The model under review builds one solid part; all positions refer to its coordinate system, in mm. A direction names the side the tool comes from. Round coordinates to 2 decimals unless told otherwise and drop trailing zeros. Order: outer loops, then holes, each group sorted by start corner. A loop starts at its lowest first (then second) coordinate and runs counter-clockwise, first axis right, second up. Notation, with made-up numbers: M 76.25,82 L 115.25,82 A22 ccw 115.25,109 Z; hole C 51.25,68.25 d9. An arc over 180 degrees is marked long. Answer as CSV lines item,"result". Start each with the question number.
from build123d import *

# Parameters (mm, degrees)
SKETCH_1_W          = 140
SKETCH_1_H          = 75
EXTRUDE_1_DEPTH     = 3
SKETCH_2_R          = 1.55
CUT_EXTRUDE_1_DEPTH = 3
SKETCH_3_W          = 5
SKETCH_3_H          = 55
EXTRUDE_2_DEPTH     = 15
SKETCH_5_R          = 1.55
CUT_EXTRUDE_2_DEPTH = 15
SKETCH_6_R          = 1.55
CUT_EXTRUDE_3_DEPTH = 15
FILLET_1_R          = 2
FILLET_2_R          = 1


with BuildPart() as part:
    # 草图1 → 凸台-拉伸1 (new body)
    with BuildSketch(Plane(origin=(0, 0, 0), x_dir=(1, 0, 0), z_dir=(0, 1, 0))):
        Rectangle(SKETCH_1_W, SKETCH_1_H)
    extrude(amount=EXTRUDE_1_DEPTH)

    # 草图2 → 切除-拉伸1 (cut)
    with BuildSketch(Plane.XZ):
        with Locations(Location((-49, 0, 0), (0, 0, 270))):
            Circle(SKETCH_2_R)
        with Locations(Location((-49, -30, 0), (0, 0, 270))):
            Circle(SKETCH_2_R)
        with Locations(Location((-49, 30, 0), (0, 0, 270))):
            Circle(SKETCH_2_R)
        with Locations(Location((49, 30, 0), (0, 0, 270))):
            Circle(SKETCH_2_R)
        with Locations(Location((49, 0, 0), (0, 0, 270))):
            Circle(SKETCH_2_R)
        with Locations(Location((49, -30, 0), (0, 0, 270))):
            Circle(SKETCH_2_R)
    extrude(amount=-CUT_EXTRUDE_1_DEPTH, mode=Mode.SUBTRACT)

    # 草图3 → 凸台-拉伸2 (add)
    with BuildSketch(Plane.XZ):
        with Locations((-59.5, 0)):
            Rectangle(SKETCH_3_W, SKETCH_3_H)
        with Locations((59.5, 0)):
            Rectangle(SKETCH_3_W, SKETCH_3_H)
    extrude(amount=EXTRUDE_2_DEPTH)

    # 草图5 → 切除-拉伸2 (cut)
    with BuildSketch(Plane.XZ):
        with Locations(Location((-66, 20, 0), (0, 0, 270))):
            Circle(SKETCH_5_R)
        with Locations(Location((-66, 10, 0), (0, 0, 270))):
            Circle(SKETCH_5_R)
        with Locations(Location((-66, 0, 0), (0, 0, 270))):
            Circle(SKETCH_5_R)
        with Locations(Location((-66, -10, 0), (0, 0, 270))):
            Circle(SKETCH_5_R)
        with Locations(Location((-66, -20, 0), (0, 0, 270))):
            Circle(SKETCH_5_R)
        with Locations(Location((66, -20, 0), (0, 0, 270))):
            Circle(SKETCH_5_R)
        with Locations(Location((66, -10, 0), (0, 0, 270))):
            Circle(SKETCH_5_R)
        with Locations(Location((66, 0, 0), (0, 0, 270))):
            Circle(SKETCH_5_R)
        with Locations(Location((66, 10, 0), (0, 0, 270))):
            Circle(SKETCH_5_R)
        with Locations(Location((66, 20, 0), (0, 0, 270))):
            Circle(SKETCH_5_R)
    extrude(amount=-CUT_EXTRUDE_2_DEPTH, mode=Mode.SUBTRACT)

    # 草图6 → 切除-拉伸3 (cut)
    with BuildSketch(Plane.ZY.offset(62)):
        with Locations((-20.625, -12.5)):
            Circle(SKETCH_6_R)
        with Locations((-13.766824394, -12.463345811)):
            Circle(SKETCH_6_R)
        with Locations((-6.911518496, -12.401024848)):
            Circle(SKETCH_6_R)
        with Locations((6.736772336, -12.494506292)):
            Circle(SKETCH_6_R)
        with Locations((13.810201603, -12.556827255)):
            Circle(SKETCH_6_R)
        with Locations((20.572026056, -12.587987736)):
            Circle(SKETCH_6_R)
    cut_extrude_3 = extrude(amount=-CUT_EXTRUDE_3_DEPTH, mode=Mode.SUBTRACT)

    # 镜向1: 切除-拉伸3 across plane
    add(cut_extrude_3.mirror(Plane(origin=(0, 0, 0), x_dir=(0, 0, 1), z_dir=(1, 0, 0))), mode=Mode.SUBTRACT)

    # 圆角1
    fillet_1_edges = [part.edges().sort_by_distance(p)[0] for p in [
        (70, 1.5, 37.5),
        (70, 1.5, -37.5),
        (-70, 1.5, -37.5),
        (-70, 1.5, 37.5),
    ]]
    fillet(fillet_1_edges, radius=FILLET_1_R)

    # 圆角2
    fillet_2_edges = [part.edges().sort_by_distance(p)[0] for p in [
        (-59.5, 0, 27.5),
        (-62, 0, 0),
        (-59.5, 0, -27.5),
        (-57, 0, 0),
        (-59.5, -15, 27.5),
        (-59.5, -15, -27.5),
        (59.5, 0, -27.5),
        (62, 0, 0),
        (59.5, 0, 27.5),
        (57, 0, 0),
        (59.5, -15, -27.5),
        (59.5, -15, 27.5),
    ]]
    fillet(fillet_2_edges, radius=FILLET_2_R)


solid = part.part
Item 1: For pin 1 (1.9 mm diameter, centred on x = -66, z = 20, fed in from +Y); pin 2 (4 mm diameter, centred on x = -49, z = -30, fed in from -Y); pin 3 (3.5 mm diameter, centred on y = -12.56, z = 13.81, fed in from -X); pin 4 (4 mm diameter, centred on x = -59, y = -9.5, fed in from -Z), all flat-tipped, find the tip position at first contact; note any pin that passes through.
Item 2: Wall thickness on probe 1 along Z at (x, y) = (-66, 2.15); probe 2 along X at (y, z) = (1, 0); probe 3 along X at (y, z) = (1.8, 30): over which ranges is each line inside the solid? List them lowest first. Write a range as [from, to].
Item 3: Consider section C-C (z = 10). State the section outline as (x, y) points, and give its area (3 significant figures).
Item 4: Consider section D-D (x = 49). State the section outline as (y, z) points.
Item 5: The part is to be moulded in two halves that separate along Y. For faces 4 (the flat face through (-1, 3, -1)), 5 (the flat face through (-57, -8, 0)), 6 (the cylindrical face through (-59.535, -11.281, 21.405)), say which applies: +Y half, -Y half, draft (parallel to the pull), parting line (faces both ways), or undercut.
Item 6: Consider section A-A (x = 66). State the section outline as (y, z) points.
Item 7: Tool access review of faces 1 (the flat face through (-62, -8, 0)), 2 (the flat face through (-60, -7, -27.5)), 3 (the flat face through (-60, -7, 27.5)): name each direction out of +Z, -Z, +X, -X, +Y, -Y from which nothing blocks a thin tool from reaching the whole face with its end or side.
Item 8: Consider section B-B (y = -7.25). State the section outline as (x, z) points, and give its area (3 significant figures).
Reported:
1,pin 1,"passes through"
1,pin 2,"stops at y = 0"
1,pin 3,"stops at x = -62"
1,pin 4,"stops at z = -27.5"
2,probe 1,"z = [-37.5, -21.55], [-18.45, -11.55], [-8.45, -1.55], [1.55, 8.45], [11.55, 18.45], [21.55, 37.5]"
2,probe 2,"x = [-70, -67.55], [-64.45, -50.55], [-47.45, 47.45], [50.55, 64.45], [67.55, 70]"
2,probe 3,"x = [-70, -50.55], [-47.45, 47.45], [50.55, 70]"
3,outline,"M -70,0 L -67.55,0 L -67.55,3 L -70,3 Z; M -64.45,0 L -63,0 A1 cw -62,-1 L -62,-15 L -57,-15 L -57,-1 A1 cw -56,0 L 56,0 A1 cw 57,-1 L 57,-15 L 62,-15 L 62,-1 A1 cw 63,0 L 64.45,0 L 64.45,3 L -64.45,3 Z; M 67.55,0 L 70,0 L 70,3 L 67.55,3 Z"
3,area,"552 mm²"
4,outline,"M 0,-37.5 L 3,-37.5 L 3,-31.55 L 0,-31.55 Z; M 0,-28.45 L 3,-28.45 L 3,-1.55 L 0,-1.55 Z; M 0,1.55 L 3,1.55 L 3,28.45 L 0,28.45 Z; M 0,31.55 L 3,31.55 L 3,37.5 L 0,37.5 Z"
5,face 4,"+Y half"
5,face 5,"draft"
5,face 6,"undercut"
6,outline,"M 0,-37.5 L 3,-37.5 L 3,-21.55 L 0,-21.55 Z; M 0,-18.45 L 3,-18.45 L 3,-11.55 L 0,-11.55 Z; M 0,-8.45 L 3,-8.45 L 3,-1.55 L 0,-1.55 Z; M 0,1.55 L 3,1.55 L 3,8.45 L 0,8.45 Z; M 0,11.55 L 3,11.55 L 3,18.45 L 0,18.45 Z; M 0,21.55 L 3,21.55 L 3,37.5 L 0,37.5 Z"
7,face 1,"+Z, -Z, -X, -Y"
7,face 2,"-Z, +X, -X, -Y"
7,face 3,"+Z, +X, -X, -Y"
8,outline,"M -62,-27.5 L -57,-27.5 L -57,27.5 L -62,27.5 Z; M 57,-27.5 L 62,-27.5 L 62,27.5 L 57,27.5 Z"
8,area,"550 mm²"
